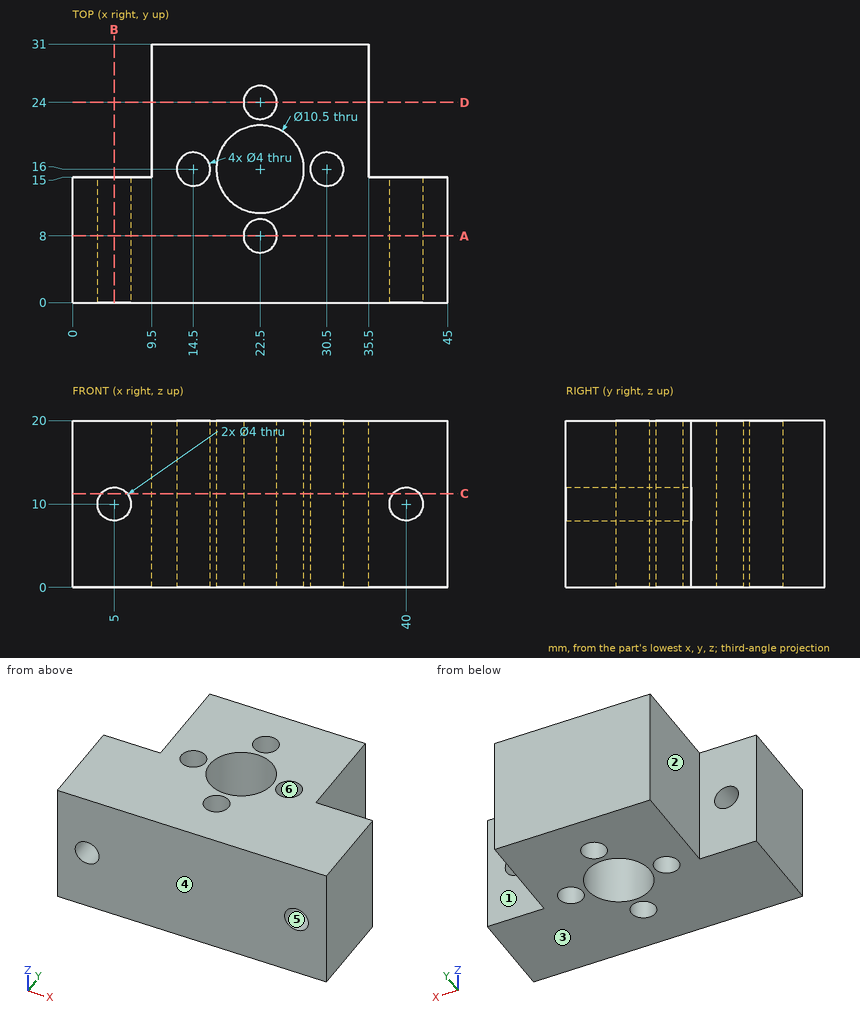
Geometry check sheet. Reference: drawing and pictorial views, mm from the part's lowest x, y, z. A direction names the side the tool comes from. Coordinates: 2 decimals unless noted, no trailing zeros. Write each loop counter-clockwise with the first axis right and the second up, starting at its lowest first coordinate (ties: lowest second). Pieces come first, ordered by that corner, then holes. Notation, with made-up numbers: (-16.5, 74) -> (1.5, 74) arc R10 cw to (1.5, 83) -> close; hole circle Ø8 at (12.25, 80.25). An arc over 180 degrees is marked (long way). One line per question, with ' | ' between items.
1. Cross-section at A-A on y = 8. Record the cut outline in (x, z).
Answers:
outline: (0, 0) -> (20.5, 0) -> (20.5, 20) -> (0, 20) -> close; (24.5, 0) -> (45, 0) -> (45, 20) -> (24.5, 20) -> close; hole circle Ø4 at (5, 10); hole circle Ø4 at (40, 10)
2. Cross-section at C-C on z = 11.25. Record the cut outline in (x, y), and give its area (3 significant figures).
Answers:
outline: (0, 0) -> (3.44, 0) -> (3.44, 15) -> (0, 15) -> close; (6.56, 0) -> (38.44, 0) -> (38.44, 15) -> (35.5, 15) -> (35.5, 31) -> (9.5, 31) -> (9.5, 15) -> (6.56, 15) -> close; (41.56, 0) -> (45, 0) -> (45, 15) -> (41.56, 15) -> close; hole circle Ø4 at (14.5, 16); hole circle Ø10.5 at (22.5, 16); hole circle Ø4 at (22.5, 8); hole circle Ø4 at (22.5, 24); hole circle Ø4 at (30.5, 16) | area: 860 mm²
3. Depth check by flat-ended pin: pin 1 Ø2.5 at (x, y) = (22.5, 8) entering from +Z; pin 2 Ø8 at (y, z) = (22.5, 12) entering from -X; pin 3 Ø1 at (x, z) = (37, 7.5) entering from +Y. Enter the tip coordinate at first touch or a pass-through.
Answers:
pin 1: passes through | pin 2: stops at x = 9.5 | pin 3: stops at y = 15
4. Cross-section at B-B on x = 5. Record the cut outline in (y, z).
Answers:
outline: (0, 0) -> (15, 0) -> (15, 8) -> (0, 8) -> close; (0, 12) -> (15, 12) -> (15, 20) -> (0, 20) -> close
5. Cross-section at D-D on y = 24. Record the cut outline in (x, z).
Answers:
outline: (9.5, 0) -> (20.5, 0) -> (20.5, 20) -> (9.5, 20) -> close; (24.5, 0) -> (35.5, 0) -> (35.5, 20) -> (24.5, 20) -> close
6. Thickness scan on probe 1 along Y at (x, z) = (22.5, 9.5); probe 2 along Y at (x, z) = (14.5, 8.25); probe 3 along Y at (x, z) = (23, 10.5). Record the ranges inside material, lowest first. Write a range as from..to.
Answers:
probe 1: y = 0..6, 10..10.75, 21.25..22, 26..31 | probe 2: y = 0..14, 18..31 | probe 3: y = 0..6.06, 9.94..10.77, 21.23..22.06, 25.94..31
7. Set-up check for the marked faces 1, 2 and 3: record each of +Z, -Z, +X, -X, +Y, -Y from which the full face is reachable in a straight line by a thin tool's end or side.
Answers:
face 1: +Z, -Z, +X, +Y | face 2: +Z, -Z, -X, +Y | face 3: -Z, +X, -X, +Y, -Y
8. Draft check along Y on the marked faces 4, 5 and 6. Enter one of: +Y half, -Y half, draft (parallel to the pull), parting line (faces both ways), or undercut.
Answers:
face 4: -Y half | face 5: draft | face 6: undercut
